```python
from build123d import *

# Parameters (mm, degrees)
F0_R     = 69.85
F1_DEPTH = 25.4
F2_R     = 66.675
F3_DEPTH = 15.875
F4_R     = 1.1303
F5_DEPTH = 5.08


with BuildPart() as f1:
    # F0 (on Top) → F1 (new body)
    with BuildSketch(Plane.XY):
        Circle(F0_R)
    extrude(amount=F1_DEPTH)

    # F2 (on face) → F3 (cut)
    with BuildSketch(Plane.XY.offset(25.4)):
        Circle(F2_R)
    extrude(amount=-F3_DEPTH, mode=Mode.SUBTRACT)

    # F4 (on face) → F5 (cut)
    with BuildSketch(Plane(origin=(0, 0, 0), x_dir=(1, 0, 0), z_dir=(0, 0, -1))):
        with Locations((0, 38.1)):
            Circle(F4_R)
        with Locations((-32.995568, 19.05)):
            Circle(F4_R)
        with Locations((-32.995568, -19.05)):
            Circle(F4_R)
        with Locations((0, -38.1)):
            Circle(F4_R)
        with Locations((32.995568, -19.05)):
            Circle(F4_R)
        with Locations((32.995568, 19.05)):
            Circle(F4_R)
    extrude(amount=-F5_DEPTH, mode=Mode.SUBTRACT)


solid = f1.part
```
CAD build for the part. Positions are in the model's coordinates, mm. Round coordinates to 2 decimals unless told otherwise and drop trailing zeros. Order: outer loops, then holes, each group sorted by start corner. A loop starts at its lowest first (then second) coordinate and runs counter-clockwise, first axis right, second up.
Q1. Slice it at A-A (y = 0). Write the cut outline in (x, z) (3 decimals).
Q2. Two-plate mould, pull along X, no slides. Class faces 1 (the flat face through (62, -26, 25.4)), 2 (the cylindrical face through (63.596, 20.027, 17.574)), 3 (the cylindrical face through (-55.431, -42.503, 12.522)), 4 (the flat face through (-1, 1, 9.525)): pulls with the +X half, pulls with the -X half, needs draft (parallel to the pull), parting line crosses it, or undercut.
Q3. Drop flat-ended pins along their axis: pin 1 (5 mm diameter, centred on y = 19.5, z = 13, fed in from -X); pin 2 (10 mm diameter, centred on x = -44.5, z = 12.5, fed in from -Y); pin 3 (10 mm diameter, centred on y = -10, z = 19, fed in from -X). Give the stop position or say it passes through.
Q4. Slice it at C-C (x = 58). Write the cut outline in (y, z) (3 decimals).
Q5. Wall check: L1, parallel to X at y = -19.05, z = 3.5; L2, parallel to Z at x = 25, y = 8 (3 decimals); L3, parallel to Y at x = 8, z = 16.25. Give the ranges that are in metal, low to high.
Q6. Slice it at B-B (z = 19.5). Write the cut outline in (x, y) (3 decimals).
Results below:
1. outline: (-69.85, 0) - (69.85, 0) - (69.85, 25.4) - (66.675, 25.4) - (66.675, 9.525) - (-66.675, 9.525) - (-66.675, 25.4) - (-69.85, 25.4) - close
2. face 1: needs draft
2. face 2: undercut
2. face 3: parting line crosses it
2. face 4: undercut
3. pin 1: stops at x = -67.75
3. pin 2: stops at y = -57.61
3. pin 3: stops at x = -69.67
4. outline: (-38.923, 0) - (38.923, 0) - (38.923, 25.4) - (32.887, 25.4) - (32.887, 9.525) - (-32.887, 9.525) - (-32.887, 25.4) - (-38.923, 25.4) - close
5. L1: x = -67.2 to -34.13, -31.87 to 31.87, 34.13 to 67.2
5. L2: z = 0 to 9.525
5. L3: y = -69.39 to -66.19, 66.19 to 69.39
6. outline: circle Ø139.7 at (0, 0); hole circle Ø133.35 at (0, 0)
